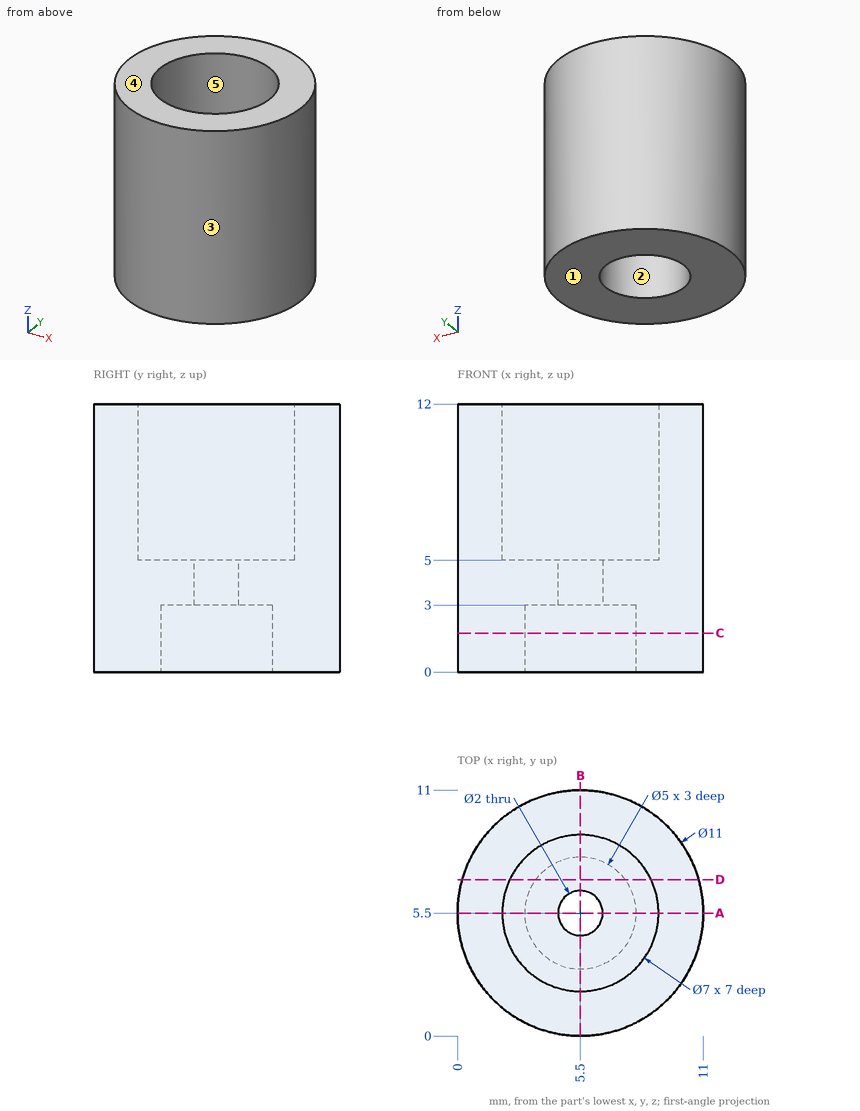
Geometry check sheet. Reference: drawing and pictorial views, mm from the part's lowest x, y, z. A direction names the side the tool comes from. Give positions to 0.01 mm unless a question says otherwise; leave off trailing zeros. Write each loop counter-clockwise with the first axis right and the second up, starting at its lowest first coordinate (ties: lowest second). Pieces come first, ordered by that corner, then holes. Notation, with made-up numbers: M 41.5,87 L 60.5,87 A19 cw 60.5,118 Z; hole C 11,-13.5 d11. An arc over 180 degrees is marked long. Put each result on its own line as item: value. Start each with the question number.
1. Scan lines: line 1 along Y through (x, z) = (5.5, 3.55); line 2 along Y through (x, z) = (5.5, 8); line 3 along Z through (x, y) = (7, 6). Record each from-to range of solid material in increasing order. Write a range as [from, to].
2. Section check A-A (y = 5.5). Record the cut outline in (x, z).
3. Go/stop test with flat-tipped pins: pin 1 Ø1.5 at (y, z) = (2, 8.5) entering from +X; pin 2 Ø2 at (y, z) = (8.5, 10) entering from -X; pin 3 Ø2 at (x, y) = (6.5, 5.5) entering from +Z. Record where each tip stops, or that it passes through.
4. Draft check along Y on the marked faces 3, 4 and 5. Enter one of: +Y half, -Y half, draft (parallel to the pull), parting line (faces both ways), or undercut.
5. Section check C-C (z = 1.75). Record the cut outline in (x, y), and give its area (3 significant figures).
6. Set-up check for the marked faces 1 and 2: record each of +Z, -Z, +X, -X, +Y, -Y from which the full face is reachable in a straight line by a thin tool's end or side.
7. Section check D-D (y = 7). Record the cut outline in (x, z).
Answer list:
1. line 1: [0, 4.5], [6.5, 11]
1. line 2: [0, 2], [9, 11]
1. line 3: [3, 5]
2. outline: M 0,0 L 3,0 L 3,3 L 4.5,3 L 4.5,5 L 2,5 L 2,12 L 0,12 Z; M 6.5,3 L 8,3 L 8,0 L 11,0 L 11,12 L 9,12 L 9,5 L 6.5,5 Z
3. pin 1: x = 10.26
3. pin 2: x = 0.38
3. pin 3: z = 5
4. face 3: parting line
4. face 4: draft
4. face 5: undercut
5. outline: C 5.5,5.5 d11; hole C 5.5,5.5 d5
5. area: 75.4 mm2
6. face 1: -Z, +X, -X, +Y, -Y
6. face 2: -Z
7. outline: M 0.21,0 L 3.5,0 L 3.5,3 L 7.5,3 L 7.5,0 L 10.79,0 L 10.79,12 L 8.66,12 L 8.66,5 L 2.34,5 L 2.34,12 L 0.21,12 Z
